```python
from build123d import *

# Parameters (mm, degrees)
F0_R     = 18.876469
F0_W     = 76.189078
F0_H     = 76.160066
F1_DEPTH = 76.2
F2_R     = 18.876469
F3_DEPTH = 31.496


with BuildPart() as f1:
    # F0 (on Front) → F1 (new body)
    with BuildSketch(Plane.XZ):
        Polygon((76.189078, 76.495655), (-76.260686, 76.495655), (-76.260686, 0), (0, 0), (76.189078, 0), align=None)
        with Locations((-39.615575, 39.702263)):
            Circle(F0_R, mode=Mode.SUBTRACT)
        with Locations((38.094539, -38.080033)):
            Rectangle(F0_W, F0_H)
    extrude(amount=F1_DEPTH)

    # F2 (on Right) → F3 (cut)
    with BuildSketch(Plane.YZ):
        with Locations((-37.08962, -40.110841)):
            Circle(F2_R)
    extrude(amount=F3_DEPTH, mode=Mode.SUBTRACT)


solid = f1.part
```
CAD build for the part. Positions are in the model's coordinates, mm. A direction names the side the tool comes from. Coordinates: 2 decimals unless noted, no trailing zeros. Order: outer loops, then holes, each group sorted by start corner. A loop starts at its lowest first (then second) coordinate and runs counter-clockwise, first axis right, second up. Notation, with made-up numbers: (-11.5, 80) -> (-0.5, 80) arc R35 cw to (-0.5, 114) -> close; hole circle Ø11 at (5.25, 13.25). An arc over 180 degrees is marked (long way). Use one line per item in the form item = value. Start each with the question number.
1) Drill centre lines: L1, parallel to X at y = -66.5, z = 39.5; L2, parallel to X at y = -46, z = -58.5; L3, parallel to Z at x = -20, y = -23.5. Where is each one in solid material? Low to high. Write a range as [from, to].
2) Band-saw the part on B-B on x = -47.5. Give the cut face in (y, z).
3) Band-saw the part on C-C on y = -22. Give the cut face in (x, z), then the cut area to 3 significant figures.
4) Tool access for faces 4 (the flat face through (-39, -38, 0)), 5 (the cylindrical face through (15.53, -51, -27.35)), 6 (the flat face through (1, -38, 76.496)): list every direction of +Z, -Z, +X, -X, +Y, -Y with a clear straight run to the whole face (end or side of a thin tool).
5) Pull direction X, two halves, no side cores. Call faces 1 (the cylindrical face through (-43.708, -37.567, 21.275)), 2 (the flat face through (0, -46, -22)), 3 (the flat face through (38, -38, -76.16)): +X half, -X half, draft (parallel to the pull), parting line (faces both ways), or undercut.
6) Band-saw the part on A-A on z = 30. Give the cut face in (x, y).
7) Drop flat-ended pins along their axis: pin 1 (19 mm diameter, centred on y = -35.5, z = -33, fed in from -X); pin 2 (1 mm diameter, centred on y = -53.5, z = -27.5, fed in from -X). Give the stop position or say it passes through.
8) Band-saw the part on D-D on x = 7. Give the cut face in (y, z).
Entries:
q1.L1 = [-76.26, -58.49], [-20.74, 76.19]
q1.L2 = [0, 76.19]
q1.L3 = [0, 76.5]
q2.outline = (-76.2, 0) -> (0, 0) -> (0, 22.55) -> (-76.2, 22.55) -> close; (-76.2, 56.85) -> (0, 56.85) -> (0, 76.5) -> (-76.2, 76.5) -> close
q3.outline = (-76.26, 0) -> (0, 0) -> (0, -28.77) -> (31.5, -28.77) -> (31.5, -51.45) -> (0, -51.45) -> (0, -76.16) -> (76.19, -76.16) -> (76.19, 76.5) -> (-76.26, 76.5) -> close; hole circle Ø37.75 at (-39.62, 39.7)
q3.area = 15,600 mm2
q4.face_4 = -Z, -X, +Y, -Y
q4.face_5 = -X
q4.face_6 = +Z, +X, -X, +Y, -Y
q5.face_1 = undercut
q5.face_2 = -X half
q5.face_3 = draft
q6.outline = (-76.26, -76.2) -> (-55.81, -76.2) -> (-55.81, 0) -> (-76.26, 0) -> close; (-23.42, -76.2) -> (76.19, -76.2) -> (76.19, 0) -> (-23.42, 0) -> close
q7.pin_1 = 31.5
q7.pin_2 = 0
q8.outline = (-76.2, -76.16) -> (0, -76.16) -> (0, 76.5) -> (-76.2, 76.5) -> close; hole circle Ø37.75 at (-37.09, -40.11)
